Verification items for this drawing (mm, ordinates from the low corner). Give positions to 0.01 mm unless a question says otherwise; leave off trailing zeros. Order: outer loops, then holes, each group sorted by start corner. A loop starts at its lowest first (then second) coordinate and runs counter-clockwise, first axis right, second up. Notation, with made-up numbers: M -19,75 L 30,75 A16 ccw 30,80 Z; hole C -10,14.5 d8. An arc over 180 degrees is marked long. Return JSON: item names as keys, results as strings. Group by question number.
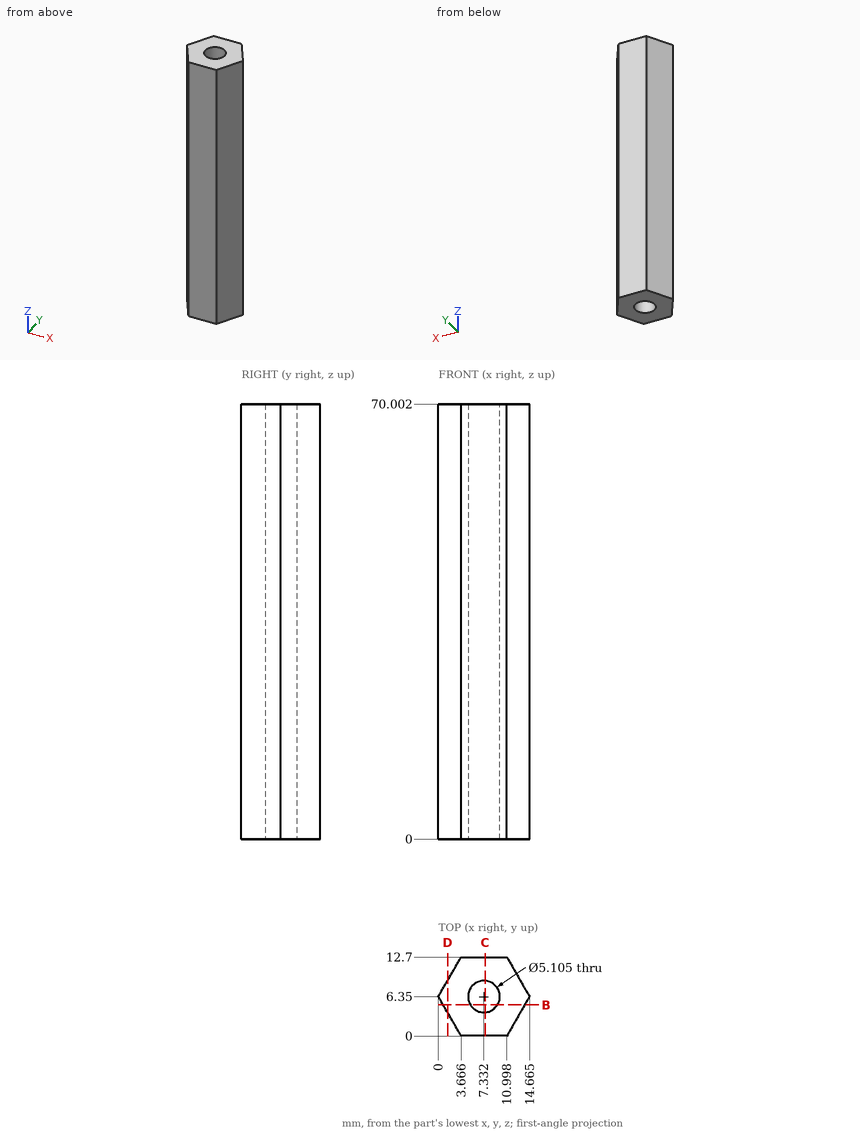
1) Sectioned sample at D-D on x = 1.5. Record the boundary of the cut face in (y, z), then the cut area to 3 significant figures.
2) Material ranges on line 1 along Y through (x, z) = (6.5, 11); line 2 along Y through (x, z) = (8.25, 9); line 3 along Y through (x, z) = (1, 47) (1 decimal), recorded low to high.
3) Depth check by flat-ended pin: P1, Ø4, axis at x = 6.5, y = 1.5, coming from the -Z side; P2, Ø3, axis at y = 2.5, z = 39, coming from the -X side; P3, Ø5, axis at y = 1.5, z = 35, coming from the +X side; P4, Ø6, axis at y = 11.5, z = 10, coming from the -X side. Enter the tip coordinate at first touch or a pass-through.
4) Sectioned sample at B-B on y = 5. Record the boundary of the cut face in (x, z) (1 decimal), then the cut area to 3 significant figures.
5) Sectioned sample at C-C on x = 7.5. Record the boundary of the cut face in (y, z).
Reply:
{
 "1": {"outline": "M 3.75,0 L 8.95,0 L 8.95,70 L 3.75,70 Z", "area": "364 mm^2"},
 "2": {"line 1": "0 to 3.94, 8.76 to 12.7", "line 2": "0 to 3.97, 8.73 to 12.7", "line 3": "4.6 to 8.1"},
 "3": {"P1": "z = 0", "P2": "x = 1.36", "P3": "x = 13.31", "P4": "x = 1.24"},
 "4": {"outline": "M 0.8,0 L 5.2,0 L 5.2,70 L 0.8,70 Z; M 9.5,0 L 13.9,0 L 13.9,70 L 9.5,70 Z", "area": "614 mm^2"},
 "5": {"outline": "M 0,0 L 3.8,0 L 3.8,70 L 0,70 Z; M 8.9,0 L 12.7,0 L 12.7,70 L 8.9,70 Z"}
}
